from build123d import *

# Parameters (mm, degrees)
BOSS_EXTRUDE1_DEPTH     = 38
CUT_EXTRUDE1_REACH      = 43.037
SKETCH2_R               = 2.15
CUT_EXTRUDE4_DEPTH      = 42.036691991
CUT_EXTRUDE4_DEPTH_BACK = 42.036691991
SKETCH3_W               = 18
SKETCH3_H               = 1
SKETCH3_H_2             = 4.881241343


with BuildPart() as part:
    # Sketch1 → Boss-Extrude1 (new body)
    with BuildSketch(Plane.XY):
        with BuildLine():
            Line((0.8, -0.368758657), (0.8, 15.131241343))
            Line((0.8, 15.131241343), (0, 15.131241343))
            Line((0, 15.131241343), (0, 0))
            ThreePointArc((0, 0), (-0.08085497, -0.393919299), (-0.310344828, -0.724137931))
            ThreePointArc((-0.310344828, -0.724137931), (2.474900525, -5.062251314), (1.5, 0))
            Line((1.5, 0), (1.5, -0.8))
            ThreePointArc((1.5, -0.8), (2.079032119, -4.355707025), (0.401769912, -1.167428159))
            ThreePointArc((0.401769912, -1.167428159), (0.69492176, -0.814981745), (0.8, -0.368758657))
        make_face()
    extrude(amount=BOSS_EXTRUDE1_DEPTH)

    # Sketch2 → Cut-Extrude1 (cut, up to next)
    with BuildSketch(Plane(origin=(0.8, 0, 0), x_dir=(0, 0, -1), z_dir=(1, 0, 0)), mode=Mode.PRIVATE) as cut_extrude1_sk1:
        with Locations((-30.5, 7.381241343)):
            Circle(SKETCH2_R)
    cut_extrude1_tool1 = extrude(cut_extrude1_sk1.sketch, amount=-CUT_EXTRUDE1_REACH, mode=Mode.PRIVATE) & part.part
    # Sketch2 → Cut-Extrude1 (cut, up to next)
    with BuildSketch(Plane(origin=(0.8, 0, 0), x_dir=(0, 0, -1), z_dir=(1, 0, 0)), mode=Mode.PRIVATE) as cut_extrude1_sk2:
        with Locations((-7.5, 7.381241343)):
            Circle(SKETCH2_R)
    cut_extrude1_tool2 = extrude(cut_extrude1_sk2.sketch, amount=-CUT_EXTRUDE1_REACH, mode=Mode.PRIVATE) & part.part
    add(cut_extrude1_tool1.solids().sort_by_distance((0.8, 7.381241, 30.5))[0], mode=Mode.SUBTRACT)
    add(cut_extrude1_tool2.solids().sort_by_distance((0.8, 7.381241, 7.5))[0], mode=Mode.SUBTRACT)

    # Sketch3 → Cut-Extrude4 (cut, two sides: drawn at the far end of the back side and taken through both)
    with BuildSketch(Plane(origin=(0.8, 0, 0), x_dir=(0, 0, -1), z_dir=(1, 0, 0)).offset(-CUT_EXTRUDE4_DEPTH_BACK)):
        with Locations((-19, 0.131241343)):
            Rectangle(SKETCH3_W, SKETCH3_H)
        with Locations((-19, -2.809379328)):
            Rectangle(SKETCH3_W, SKETCH3_H_2)
    extrude(amount=CUT_EXTRUDE4_DEPTH + CUT_EXTRUDE4_DEPTH_BACK, mode=Mode.SUBTRACT)


solid = part.part
Input: part model. Units: mm. Frame: model coordinates. A direction names the side the tool comes from. Give positions to 0.01 mm unless a question says otherwise; leave off trailing zeros. Loops run counter-clockwise (first coordinate to the right, second up) from the corner with the lowest first, then second, coordinate; pieces in that order, holes last. Notation, with made-up numbers: (-27.5, 31.25) - (-0.5, 31.25) arc R24 cw to (-0.5, 53.25) - close; hole circle Ø8 at (-16.5, 78.5). An arc over 180 degrees is marked (long way). Use CSV: the item, a comma, the result in double quotes. Start each with the question number.
Item 1: Mould query, pull axis Z, two halves, no side actions, for faces 6 (the flat face through (0.8, 7, 19)), 7 (the cylindrical face through (0.41, 8.03, 5.45)), 8 (the flat face through (0.5, 2.7, 0)). Classes: pulls with the +Z half, pulls with the -Z half, needs draft (parallel to the pull), parting line crosses it, or undercut.
Item 2: Section B-B on y = -3.25. Return loops of the section in (x, z).
Item 3: Contact query for flat-ended pins moving along their axis: P1, Ø3, axis at x = 1.5, y = -2.625, coming from the +Z side; P2, Ø4.5, axis at y = 10.5, z = 16.5, coming from the +X side; P3, Ø4.5, axis at y = 7.5, z = 21, coming from the -X side; P4, Ø8, axis at y = 0.5, z = 13, coming from the -X side. Output: stop coordinate, or through.
Item 4: Reachability of faces 1 (the flat face through (0, 8, 19)), 2 (the flat face through (1.5, -0.4, 32.9)), 3 (the flat face through (0.5, 2.7, 38)), 4 (the cylindrical face through (2.15, -4.33, 4.93)), 5 (the flat face through (0, -4, 10)) from +Z, -Z, +X, -X, +Y, -Y: full face, straight path, thin tool, end or side. Return the list, or none.
Item 5: Section C-C on z = 4. Return loops of the section in (x, y) (3 decimals), then the cut area to 3 significant figures.
Item 6: Line query: line 1 (Y direction, x = 0.2, z = 30.5); line 2 (Z direction, x = -0.05, y = -4.5); line 3 (Y direction, x = 0.5, z = 7.5). Output: solid intervals per line, ascending.
Item 7: Section A-A on z = 30.5. Return loops of the section in (x, y) (3 decimals).
Item 8: Section D-D on y = 6.25. Return loops of the section in (x, z), then the cut area to 3 significant figures.
Ans:
1,face 6,"needs draft"
1,face 7,"undercut"
1,face 8,"pulls with the -Z half"
2,outline,"(-1.05, 0) - (-0.21, 0) - (-0.21, 10) - (-1.05, 10) - close; (-1.05, 28) - (-0.21, 28) - (-0.21, 38) - (-1.05, 38) - close; (3.21, 0) - (4.05, 0) - (4.05, 10) - (3.21, 10) - close; (3.21, 28) - (4.05, 28) - (4.05, 38) - (3.21, 38) - close"
3,P1,"passes through"
3,P2,"stops at x = 0.8"
3,P3,"stops at x = 0"
3,P4,"stops at x = -1.08"
4,face 1,"+Z, -Z, -X, +Y"
4,face 2,"+Z, -Z, +Y"
4,face 3,"+Z, +X, -X, +Y, -Y"
4,face 4,"+Z, -Z"
4,face 5,"+X, -X, -Y"
5,outline,"(-0.31, -0.724) arc R2.625 ccw (long way) to (1.5, 0) - (1.5, -0.8) arc R1.825 cw (long way) to (0.402, -1.167) arc R1 ccw to (0.8, -0.369) - (0.8, 15.131) - (0, 15.131) - (0, 0) arc R1 cw to start"
5,area,"22.9 mm2"
6,line 1,"y = -4.91 to -3.91, -1.34 to 5.23, 9.53 to 15.13"
6,line 2,"z = 0 to 10, 28 to 38"
6,line 3,"y = -5.05 to -4.15, -1.08 to 5.23, 9.53 to 15.13"
7,outline,"(-0.31, -0.724) arc R2.625 ccw (long way) to (1.5, 0) - (1.5, -0.8) arc R1.825 cw (long way) to (0.402, -1.167) arc R1 ccw to (0.8, -0.369) - (0.8, 5.231) - (0, 5.231) - (0, 0) arc R1 cw to start; (0, 9.531) - (0.8, 9.531) - (0.8, 15.131) - (0, 15.131) - close"
8,outline,"(0, 0) - (0.8, 0) - (0.8, 5.67) - (0, 5.67) - close; (0, 9.33) - (0.8, 9.33) - (0.8, 28.67) - (0, 28.67) - close; (0, 32.33) - (0.8, 32.33) - (0.8, 38) - (0, 38) - close"
8,area,"24.5 mm2"
